Here's how the part is built. I have some questions about the finished solid (model axes, mm). A direction names the side the tool comes from. Coordinates: 2 decimals unless noted, no trailing zeros. Write each loop counter-clockwise with the first axis right and the second up, starting at its lowest first coordinate (ties: lowest second). Pieces come first, ordered by that corner, then holes. Notation, with made-up numbers: (19.25, 8.25) - (38.25, 8.25) arc R26 ccw to (38.25, 27.25) - close; hole circle Ø6 at (26.5, 76.5). An arc over 180 degrees is marked (long way). Answer in a Markdown table with one row per item. Add a question column.
Item 1: Imagine slicing it at B-B (z = 0). Please give me the cut outline in (x, y).
Item 2: Which directions (+Z, -Z, +X, -X, +Y, -Y) give clear straight access to the entire face, cutting with the end or side of a thin tool? Please do faces 4 (the face through (5, -6, 0)), 5 (the face through (6.06, -2.28, 2.98)).
Item 3: If I drill on probe 1 along Y at (x, z) = (7.5, 0); probe 2 along Y at (x, z) = (1.6, 0); probe 3 along X at (y, z) = (-1, 2.75), over which ranges is the centre line in solid material (lowest first)? Write a range as from..to.
Item 4: Imagine slicing it at C-C (z = 2.25). Please give me the cut outline in (x, y).
Item 5: Imagine slicing it at A-A (x = 7). Please give me the cut outline in (y, z), plus the area to 3 significant figures.
Item 6: Imagine slicing it at D-D (y = -4). Please give me the cut outline in (x, z), plus the area to 3 significant figures.
Item 7: We'd pull the mould along Z, two halves only. Please class faces 1 (the face through (1.01, 0.07, 1.5)), 2 (the face through (10, 3, -3)), 3 (the face through (4.93, -3.042, -5.172)): +Z half, -Z half, draft (parallel to the pull), parting line (faces both ways), or undercut.
Item 8: I'm going to push a flat-ended pin straight in: pin 1 (1.5 mm diameter, centred on x = 3, z = 4, fed in from +Y). Where does the tip first touch, or does it pass through?
from build123d import *

# Parameters (mm, degrees)
EXTRUDE_1_DEPTH     = 10
SKETCH_2_R          = 3.75277675
CUT_EXTRUDE_1_DEPTH = 8
SKETCH_3_R          = 1.5
CUT_EXTRUDE_2_DEPTH = 7


with BuildPart() as part:
    # 草图1 → 凸台-拉伸1 (new body)
    with BuildSketch(Plane(origin=(0, 0, 0), x_dir=(0, 0, -1), z_dir=(1, 0, 0))):
        Polygon((6.92820323, 0), (3.464101615, 6), (-3.464101615, 6), (-6.92820323, 0), (-3.464101615, -6), (3.464101615, -6), align=None)
    extrude(amount=EXTRUDE_1_DEPTH)

    # 草图2 → 切除-拉伸1 (cut)
    with BuildSketch(Plane(origin=(10, 0, 0), x_dir=(0, 0, -1), z_dir=(1, 0, 0))):
        Circle(SKETCH_2_R)
    extrude(amount=-CUT_EXTRUDE_1_DEPTH, mode=Mode.SUBTRACT)

    # 草图3 → 切除-拉伸2 (cut)
    with BuildSketch(Plane(origin=(2, 0, 0), x_dir=(0, 0, -1), z_dir=(1, 0, 0))):
        Circle(SKETCH_3_R)
    extrude(amount=-CUT_EXTRUDE_2_DEPTH, mode=Mode.SUBTRACT)


solid = part.part
Here are the results:
| question | item | result |
|---|---|---|
| 1 | outline | (0, -6) - (10, -6) - (10, -3.75) - (2, -3.75) - (2, -1.5) - (0, -1.5) - close; (0, 1.5) - (2, 1.5) - (2, 3.75) - (10, 3.75) - (10, 6) - (0, 6) - close |
| 2 | face 4 | +Z, -Z, +X, -X, -Y |
| 2 | face 5 | +X |
| 3 | probe 1 | y = -6..-3.75, 3.75..6 |
| 3 | probe 2 | y = -6..-1.5, 1.5..6 |
| 3 | probe 3 | x = 0..2 |
| 4 | outline | (0, -6) - (10, -6) - (10, -3) - (2, -3) - (2, 3) - (10, 3) - (10, 6) - (0, 6) - close |
| 5 | outline | (-6, -3.46) - (0, -6.93) - (6, -3.46) - (6, 3.46) - (0, 6.93) - (-6, 3.46) - close; hole circle Ø7.51 at (0, 0) |
| 5 | area | 80.5 mm2 |
| 6 | outline | (0, -4.62) - (10, -4.62) - (10, 4.62) - (0, 4.62) - close |
| 6 | area | 92.4 mm2 |
| 7 | face 1 | undercut |
| 7 | face 2 | draft |
| 7 | face 3 | -Z half |
| 8 | pin 1 | stops at y = 6 |
